Here's how the part is built. I have some questions about the finished solid (model axes, mm). A direction names the side the tool comes from. Give positions to 0.01 mm unless a question says otherwise; leave off trailing zeros. Loops run counter-clockwise (first coordinate to the right, second up) from the corner with the lowest first, then second, coordinate; pieces in that order, holes last. Notation, with made-up numbers: (87, -35) - (142, -35) arc R12 ccw to (142, -27) - close; hole circle Ø11 at (72.25, 50). An arc over 180 degrees is marked (long way). Return JSON: item names as keys, results as strings. Group by question number.
(1) If we section it at A-A (y = 0): Please give me the cut outline in (x, z).
(2) If we section it at B-B (x = 0): Please give me the cut outline in (y, z), then the cut area to 3 significant figures.
(3) If we section it at C-C (z = 7.75): Please give me the cut outline in (x, y), then the cut area to 3 significant figures.
(4) For P1, Ø4.5, axis at x = 25.4, y = 0, coming from the -Z side, with a flat end and sliding along its axis, tell me the tip position at first contact or that it passes through.
(5) If we section it at D-D (x = 25.4): Please give me the cut outline in (y, z).
(6) I need wall thicknesses on probe 1 along Y at (x, z) = (12.7, 4.5); probe 2 along Y at (x, z) = (-25.4, 1.5); probe 3 along Z at (x, y) = (0, 25.75). Which ranges of each line are inside material? Lowest first, please. Write a range as [from, to].
(7) If we mould it in two halves opening along X, with no side actions, what happens to faces 4 (the flat face through (-35, 0, 12)), 5 (the flat face through (-0.5, 35, 9.5)), 6 (the cylindrical face through (14.072, -19.845, 3.131))? For each: released by +X, released by -X, zero draft, split by the parting line, or undercut.
(8) On a 3-axis mill with a long thin cutter (end or side, diameter ignored), from which of +Z, -Z, +X, -X, +Y, -Y can I reach the whole of each face in a straight line? I mean faces 1 (the cylindrical face through (0.553, 20.611, 10.008)), 2 (the flat face through (35, 0, 12)), 3 (the cylindrical face through (-27.95, 0.11, 3.13)). Say none if no direction works.
```python
from build123d import *

# Parameters (mm, degrees)
F0_W     = 70
F0_H     = 70
F1_DEPTH = 25
F2_R     = 2.5527
F3_DEPTH = 6.35
F4_R     = 6.35
F5_DEPTH = 25
F6_R     = 2.5527
F7_DEPTH = 30.1856882138


with BuildPart() as f1:
    # F0 (on Top) → F1 (new body)
    with BuildSketch(Plane.XY):
        Rectangle(F0_W, F0_H)
    extrude(amount=F1_DEPTH)

    # F2 (on Top) → F3 (cut)
    with BuildSketch(Plane.XY):
        Circle(F2_R)
        with Locations((-25.4, 0)):
            Circle(F2_R)
        with Locations((-12.7, -21.9970452561)):
            Circle(F2_R)
        with Locations((12.7, -21.9970452561)):
            Circle(F2_R)
        with Locations((25.4, 0)):
            Circle(F2_R)
        with Locations((12.7, 21.9970452561)):
            Circle(F2_R)
        with Locations((-12.7, 21.9970452561)):
            Circle(F2_R)
    extrude(amount=F3_DEPTH, mode=Mode.SUBTRACT)

    # F4 (on face) → F5 (cut, through all)
    with BuildSketch(Plane.XY.offset(25)):
        Circle(F4_R)
    extrude(amount=-F5_DEPTH, mode=Mode.SUBTRACT)

    # F6 (on face) → F7 (cut, up to face)
    with BuildSketch(Plane(origin=(0, 35, 0), x_dir=(-1, 0, 0), z_dir=(0, 1, 0))):
        with Locations((0, 12.5)):
            Circle(F6_R)
    extrude(amount=-F7_DEPTH, mode=Mode.SUBTRACT)


solid = f1.part
```
Values:
{
 "1": {"outline": "(-35, 0) - (-27.95, 0) - (-27.95, 6.35) - (-22.85, 6.35) - (-22.85, 0) - (-6.35, 0) - (-6.35, 25) - (-35, 25) - close; (6.35, 0) - (22.85, 0) - (22.85, 6.35) - (27.95, 6.35) - (27.95, 0) - (35, 0) - (35, 25) - (6.35, 25) - close"},
 "2": {"outline": "(-35, 0) - (-6.35, 0) - (-6.35, 25) - (-35, 25) - close; (6.35, 0) - (35, 0) - (35, 9.95) - (6.35, 9.95) - close; (6.35, 15.05) - (35, 15.05) - (35, 25) - (6.35, 25) - close", "area": "1,290 mm2"},
 "3": {"outline": "(-35, -35) - (35, -35) - (35, 35) - (-35, 35) - close; hole circle Ø12.7 at (0, 0)", "area": "4,770 mm2"},
 "4": {"P1": "z = 6.35"},
 "5": {"outline": "(-35, 0) - (-2.55, 0) - (-2.55, 6.35) - (2.55, 6.35) - (2.55, 0) - (35, 0) - (35, 25) - (-35, 25) - close"},
 "6": {"probe 1": "[-35, -24.55], [-19.44, 19.44], [24.55, 35]", "probe 2": "[-35, -2.55], [2.55, 35]", "probe 3": "[0, 9.95], [15.05, 25]"},
 "7": {"face 4": "released by -X", "face 5": "zero draft", "face 6": "undercut"},
 "8": {"face 1": "+Y", "face 2": "+Z, -Z, +X, +Y, -Y", "face 3": "-Z"}
}
